Read the model definition and answer for the solid it produces. Units are mm, in the model's axes. A direction names the side the tool comes from. Give positions to 0.01 mm unless a question says otherwise; leave off trailing zeros. Write each loop counter-clockwise with the first axis right and the second up, starting at its lowest first coordinate (ties: lowest second). Pieces come first, ordered by that corner, then holes. Notation, with made-up numbers: (66.5, 89.5) -> (124.5, 89.5) arc R18 cw to (124.5, 98.5) -> close; hole circle Ø10 at (82.5, 58). An arc over 180 degrees is marked (long way). Write item = value, one per line.
from build123d import *

# Parameters (mm, degrees)
F0_W     = 44.8976987973
F0_H     = 31.3708279282
F1_DEPTH = 25.4
F2_W     = 44.8976987973
F2_H     = 25.4
F3_DEPTH = 25.4
F4_R     = 4.1790450116
F5_DEPTH = 25.4


with BuildPart() as f1:
    # F0 (on Top) → F1 (new body)
    with BuildSketch(Plane.XY):
        with Locations((-35.9757202677, 11.9439391419)):
            Rectangle(F0_W, F0_H)
    extrude(amount=F1_DEPTH)

    # F2 (on face) → F3 (join)
    with BuildSketch(Plane(origin=(0, 27.629353106, 0), x_dir=(-1, 0, 0), z_dir=(0, 1, 0))):
        with BuildLine():
            Line((58.4245696664, 0), (13.5268708691, 0))
            ThreePointArc((13.5268708691, 0), (35.9757202677, -17.5745007714), (58.4245696664, 0))
        make_face()
        with Locations((35.9757202677, 12.7)):
            Rectangle(F2_W, F2_H)
    extrude(amount=F3_DEPTH)

    # F4 (on face) → F5 (cut)
    with BuildSketch(Plane(origin=(0, 53.029353106, 0), x_dir=(-1, 0, 0), z_dir=(0, 1, 0))):
        with Locations((34.8900407553, -6.8504069932)):
            Circle(F4_R)
    extrude(amount=-F5_DEPTH, mode=Mode.SUBTRACT)


solid = f1.part
(1) A tool of negligible diameter and unlimited length cuts with its end or side. For faces 5 (the flat face through (-41, 27.629, -7)), 6 (the flat face through (-58.425, 24, 13)), from which of +Z, -Z, +X, -X, +Y, -Y can it reach the whole face along a straight path? Write none if from no direction.
Checks:
face_5 = -Z, +X, -X, -Y
face_6 = +Z, -Z, -X, +Y, -Y
(2) The part is cut by section A-A on z = -9. Determine the outline of the cut face in (x, y), plus the area to 3 significant figures.
Checks:
outline = (-53.95, 27.63) -> (-38.47, 27.63) -> (-38.47, 53.03) -> (-53.95, 53.03) -> close; (-31.31, 27.63) -> (-18, 27.63) -> (-18, 53.03) -> (-31.31, 53.03) -> close
area = 731 mm²
(3) For a pull along Z with two mould halves and no side action, classify faces 1 (the flat face through (-36, -3.741, 13)), 2 (the flat face through (-36, 24, 25.4)), 3 (the flat face through (-36, 12, 0)), 4 (the cylindrical face through (-31.81, 40.507, -4.026)) as released by +Z, released by -Z, zero draft, split by the parting line, or undercut.
Checks:
face_1 = zero draft
face_2 = released by +Z
face_3 = released by -Z
face_4 = undercut
(4) The part is cut by section C-C on x = -25.5. Determine the outline of the cut face in (y, z), plus the area to 3 significant figures.
Checks:
outline = (-3.74, 0) -> (27.63, 0) -> (27.63, -15.07) -> (53.03, -15.07) -> (53.03, 25.4) -> (-3.74, 25.4) -> close
area = 1,820 mm²
(5) The part is cut by section B-B on y = 28.5. Determine the outline of the cut face in (x, z), plus the area to 3 significant figures.
Checks:
outline = (-58.42, 0) arc R23.12 ccw to (-13.53, 0) -> (-13.53, 25.4) -> (-58.42, 25.4) -> close; hole circle Ø8.36 at (-34.89, -6.85)
area = 1,670 mm²
(6) Consider L1, parallel to Z at x = -53.5, y = 11.5; L2, parallel to Z at x = -32.5, y = 35.5; L3, parallel to Y at x = -45, z = -7.5. Determine where each line is inside the solid, lowest interval first.
Checks:
L1 = 0 to 25.4
L2 = -17.31 to -10.28, -3.42 to 25.4
L3 = 27.63 to 53.03
(7) The part is cut by section D-D on y = 17.5. Determine the outline of the cut face in (x, z).
Checks:
outline = (-58.42, 0) -> (-13.53, 0) -> (-13.53, 25.4) -> (-58.42, 25.4) -> close
(8) Given P1, Ø3, axis at x = -31.5, z = -6.5, coming from the -Y side; P2, Ø1.5, axis at x = -40.5, y = 9, coming from the -Z side; P3, Ø8, axis at y = 19, z = -5, coming from the +X side, each flat-ended and moving along its own axis, determine where each tip first touches the part or whether it passes through.
Checks:
P1 = 27.63
P2 = 0
P3 = through
